For this review, take the finished solid that the model builds, in its own axes (mm). Coordinates: 2 decimals unless noted, no trailing zeros. Order: outer loops, then holes, each group sorted by start corner. A loop starts at its lowest first (then second) coordinate and runs counter-clockwise, first axis right, second up.
from build123d import *

# Parameters (mm, degrees)
F0_W     = 63
F0_H     = 84
F2_DEPTH = 30
F3_D     = 30
F5_D     = 42
F5_DEPTH = 15
F5_TIP   = 12.6180729996
F7_D     = 13
F8_R     = 5


with BuildPart() as f2:
    # F0 (on Top) → F2 (new body)
    with BuildSketch(Plane.XY):
        Rectangle(F0_W, F0_H)
    extrude(amount=F2_DEPTH)

    # F3 (through all)
    with Locations(Plane(origin=(0, 0, 0), x_dir=(1, 0, 0), z_dir=(0, 0, -1))):
        with Locations((0, 0)):
            Hole(F3_D / 2)

    # F5
    with Locations(Plane(origin=(0, 0, 0), x_dir=(1, 0, 0), z_dir=(0, 0, -1))):
        with Locations((0, 0)):
            Hole(F5_D / 2, depth=F5_DEPTH)
            with Locations((0, 0, -(F5_DEPTH + F5_TIP / 2))):  # 118° drill point
                Cone(0, F5_D / 2, F5_TIP, mode=Mode.SUBTRACT)

    # F7 (through all)
    with Locations(Plane(origin=(-31.5, 0, 0), x_dir=(0, -1, 0), z_dir=(-1, 0, 0))):
        with Locations((-29, 15)):
            Hole(F7_D / 2)

    # F8
    f8_edges = [f2.edges().sort_by_distance(p)[0] for p in [
        (0, 42, 30),
    ]]
    fillet(f8_edges, radius=F8_R)


solid = f2.part
1. Clearance check with a flat-ended pin moving along its axis: pin 1 Ø8 at (x, y) = (17, -7) entering from -Z. State where the tip first meets the part, or that it passes through.
Answer below:
pin 1: stops at z = 0
2. Take a section at A-A, the plane x = 0. Give the boundary of the cut face in (y, z).
Answer below:
outline: (-42, 0) - (-21, 0) - (-21, 15) - (-15, 18.61) - (-15, 30) - (-42, 30) - close; (15, 18.61) - (21, 15) - (21, 0) - (42, 0) - (42, 25) arc R5 ccw to (37, 30) - (15, 30) - close; hole circle Ø13 at (29, 15)
3. Take a section at D-D, the plane x = 26. Give the boundary of the cut face in (y, z), plus the area to 3 significant figures.
Answer below:
outline: (-42, 0) - (42, 0) - (42, 25) arc R5 ccw to (37, 30) - (-42, 30) - close; hole circle Ø13 at (29, 15)
area: 2,380 mm2
4. Take a section at C-C, the plane y = 29. Give the boundary of the cut face in (x, z), plus the area to 3 significant figures.
Answer below:
outline: (-31.5, 0) - (31.5, 0) - (31.5, 8.5) - (-31.5, 8.5) - close; (-31.5, 21.5) - (31.5, 21.5) - (31.5, 30) - (-31.5, 30) - close
area: 1,070 mm2
5. The part is to be moulded in two halves that separate along Y. For faces 1 (the face through (-20.03, -6.31, 7.6)), 2 (the face through (0, -42, 15)), 3 (the face through (0, 40, 29)), 4 (the face through (-21.4, 0.6, 0)), say which applies: +Y half, -Y half, draft (parallel to the pull), parting line (faces both ways), or undercut.
Answer below:
face 1: undercut
face 2: -Y half
face 3: +Y half
face 4: draft
6. Take a section at B-B, the plane z = 16. Give the boundary of the cut face in (x, y), plus the area to 3 significant figures.
Answer below:
outline: (-31.5, -42) - (31.5, -42) - (31.5, 22.58) - (-31.5, 22.58) - close; (-31.5, 35.42) - (31.5, 35.42) - (31.5, 42) - (-31.5, 42) - close; hole circle Ø38.67 at (0, 0)
area: 3,310 mm2
7. To check wall thickness, follow L1, parallel to Y at x = 0, z = 14.5; L2, parallel to Y at x = 0, z = 23; L3, parallel to X at y = -13.5, z = 15. State the ranges of each line that lie inside material, in increasing order.
Answer below:
L1: y = -42 to -21, 21 to 22.52, 35.48 to 42
L2: y = -42 to -15, 15 to 42
L3: x = -31.5 to -16.09, 16.09 to 31.5
